CAD build for the part. Positions are in the model's coordinates, mm. Round coordinates to 2 decimals unless told otherwise and drop trailing zeros. Order: outer loops, then holes, each group sorted by start corner. A loop starts at its lowest first (then second) coordinate and runs counter-clockwise, first axis right, second up. Notation, with made-up numbers: (71.25, 61.25) - (87.25, 61.25) arc R21 ccw to (87.25, 88.25) - close; hole circle Ø9 at (-10.5, 17.5). An arc over 180 degrees is marked (long way). Use one line per item in the form item = value. Start each with the question number.
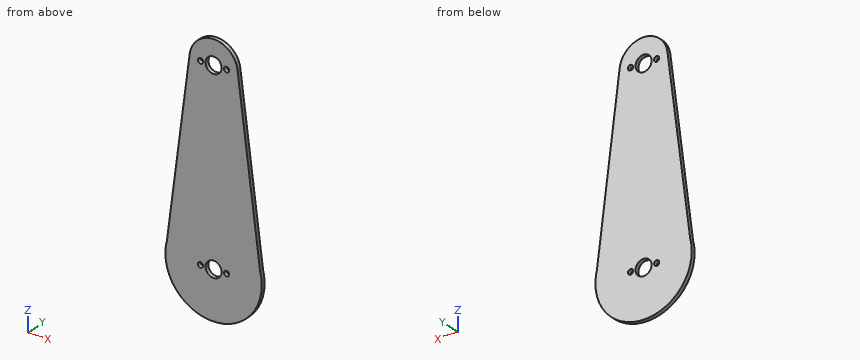
from build123d import *

# Parameters (mm, degrees)
F0_R     = 2.0828
F0_R_2   = 6.35
F1_DEPTH = 3.175


with BuildPart() as f1:
    # F0 (on Front) → F1 (new body)
    with BuildSketch(Plane.XZ):
        with BuildLine():
            Line((-36.890323, 9.524395), (-38.1, 0))
            ThreePointArc((-38.1, 0), (0, -38.1), (38.1, 0))
            Line((38.1, 0), (36.890323, 9.524395))
            ThreePointArc((36.890323, 9.524395), (0, 38.1), (-36.890323, 9.524395))
        make_face()
        with Locations((-10.31875, 0)):
            Circle(F0_R, mode=Mode.SUBTRACT)
        Circle(F0_R_2, mode=Mode.SUBTRACT)
        with Locations((10.31875, 0)):
            Circle(F0_R, mode=Mode.SUBTRACT)
        with BuildLine():
            ThreePointArc((-36.890323, 9.524395), (-37.796371, 4.800454), (-38.1, 0))
            Line((-38.1, 0), (-36.890323, 9.524395))
        make_face()
        with BuildLine():
            Line((36.890323, 9.524395), (38.1, 0))
            ThreePointArc((38.1, 0), (37.796371, 4.800454), (36.890323, 9.524395))
        make_face()
        with BuildLine():
            Line((-18.898185, 151.185483), (-36.890323, 9.524395))
            ThreePointArc((-36.890323, 9.524395), (0, 38.1), (36.890323, 9.524395))
            Line((36.890323, 9.524395), (18.898185, 151.185483))
            ThreePointArc((18.898185, 151.185483), (19.012008, 149.987768), (19.05, 148.785256))
            ThreePointArc((19.05, 148.785256), (-1.202512, 129.773248), (-18.898185, 151.185483))
        make_face()
        with BuildLine():
            ThreePointArc((18.898185, 151.185483), (0, 167.835256), (-18.898185, 151.185483))
            ThreePointArc((-18.898185, 151.185483), (-1.202512, 129.773248), (19.05, 148.785256))
            ThreePointArc((19.05, 148.785256), (19.012008, 149.987768), (18.898185, 151.185483))
        make_face()
        with Locations((-10.31875, 148.785256)):
            Circle(F0_R, mode=Mode.SUBTRACT)
        with Locations((0, 148.785256)):
            Circle(F0_R_2, mode=Mode.SUBTRACT)
        with Locations((10.31875, 148.785256)):
            Circle(F0_R, mode=Mode.SUBTRACT)
    extrude(amount=F1_DEPTH)


solid = f1.part
(1) Flat gauge pins, fed straight in: P1, Ø1, axis at x = 28.5, y = -0.5, coming from the -Z side; P2, Ø1, axis at y = -0.5, z = 35, coming from the +X side. Where does each tip first touch, or does it go through?
(2) Slice it at C-C (z = 108). Give the cut face in (x, y) (3 decimals).
(3) Wall check: line 1 (Z direction, x = -9, y = -2.95); line 2 (Z direction, x = 4, y = -2.15); line 3 (X direction, y = -2.65, z = -0.5). Give the ranges that are in metal, low to high. Write a range as [from, to].
(4) Slice it at D-D (x = 30). Give the cut face in (y, z) (3 decimals).
(5) Slice it at A-A (x = 0). Give the cut face in (y, z) (3 decimals).
(6) Slice it at B-B (y = -1.15). Give the cut face in (x, z), and give its area (3 significant figures).
Results list:
q1.P1 = -25.84
q1.P2 = 33.72
q2.outline = (-24.383, -3.175) - (24.383, -3.175) - (24.383, 0) - (-24.383, 0) - close
q3.line_1 = [-37.02, -1.61], [1.61, 147.17], [150.4, 165.58]
q3.line_2 = [-37.89, -4.93], [4.93, 143.85], [153.72, 167.41]
q3.line_3 = [-38.1, -12.34], [-8.3, -6.33], [6.33, 8.3], [12.34, 38.1]
q4.outline = (-3.175, -23.486) - (0, -23.486) - (0, 63.775) - (-3.175, 63.775) - close
q5.outline = (-3.175, -38.1) - (0, -38.1) - (0, -6.35) - (-3.175, -6.35) - close; (-3.175, 6.35) - (0, 6.35) - (0, 142.435) - (-3.175, 142.435) - close; (-3.175, 155.135) - (0, 155.135) - (0, 167.835) - (-3.175, 167.835) - close
q6.outline = (-38.1, 0) arc R38.1 ccw to (38.1, 0) arc R38.1 ccw to (36.89, 9.52) - (18.9, 151.19) arc R19.05 ccw to (-18.9, 151.19) - (-36.89, 9.52) arc R38.1 ccw to start; hole circle Ø4.17 at (-10.32, 0); hole circle Ø4.17 at (-10.32, 148.79); hole circle Ø12.7 at (0, 0); hole circle Ø12.7 at (0, 148.79); hole circle Ø4.17 at (10.32, 0); hole circle Ø4.17 at (10.32, 148.79)
q6.area = 11,100 mm²
